Autodesk Inventor part; units mm, degrees
ref_plane "Work Plane1" through (29, 0, 0) normal (0, -1, 0) x (1, 0, 0)
ref_plane "YZ Plane" through (0, 0, 0) normal (1, 0, 0) x (0, 1, 0)
ref_plane "XZ Plane" through (0, 0, 0) normal (0, 1, 0) x (-1, 0, 0)
sketch "Skizze1" plane through (0, 0, 0) normal (0, 0, 1) x (1, 0, 0)
  line L0 (-2.3333, 0) -> (20, 0)
  line L1 (20, 0) -> (20, 5)
  line L2 (20, 5) -> (3.75, 5)
  line L3 (3.75, 5) -> (2.8297, 5)
  line L4 (2.8297, 5) -> (0, 5)
  line L5 (0, 5) -> (0, 8)
  line L6 (0, 8) -> (-10, 8)
  line L7 (-10, 8) -> (-10, 4.6188)
  line L8 (-10, 4.6188) -> (-5, 4.6188)
  line L9 (-5, 4.6188) -> (-2.3333, 0)
  line L10 (-16, 0) -> (26, 0)
  line L11 (0, -1.6) -> (0, 9.6)
  line L12 (3.75, 5) -> (0, 5) construction
  dimension "d1" = 16.25
  dimension "d2" = 0.9203
  dimension "d3" = 10
  dimension "d4" = 5
  dimension "d5" = 60
  dimension "d6" = 10
  dimension "d7" = 10
  dimension "d8" = 9.2376
  dimension "d9" = 16
  dimension "d26" = 20
revolve "Körper" add sketch "Skizze1" angle 360 about axis through (-2.3333, 0, 0) along (1, 0, 0)
sketch "Skizze2" plane through (-10, 0, 0) normal (-1, 0, 0) x (0, 0, 1)
  circle A0 centre (0, 0) radius 4.6188
  line L0 (0, -11.2) -> (0, 11.2)
  line L1 (-11.2, 0) -> (11.2, 0)
  line L2 (4.6188, 0) -> (2.3094, -4)
  line L3 (2.3094, -4) -> (-2.3094, -4)
  line L4 (-2.3094, -4) -> (-4.6188, 0)
  line L5 (-4.6188, 0) -> (-2.3094, 4)
  line L6 (-2.3094, 4) -> (2.3094, 4)
  line L7 (2.3094, 4) -> (4.6188, 0)
  point P0 (0, 0)
extrude "Loch" add sketch "Skizze2" against normal up to next contours L7 A0 | A0 L2 | L6 L0 A0 | A0 L0 L3 | L0 L6 A0 | A0 L3 L0 | L4 A0 | A0 L5
fillet "Rundung1" radius 1 1 edges at (-10, -8, 0)
thread "Gewinde"
chamfer "Fase1" distance 0.9202 distance2 0.9202 1 edges at (20, -5, 0) measured on face at (20, -0.8193, -0.3214)
ref_plane "Work Plane1" through (29, 0, 0) normal (0, -1, 0) x (1, 0, 0)
fillet "Fillet2" radius 0.1 1 edges at (0, -5, 0)
equation "\"d30\" = R"
equation "\"d17\" = RR"
equation "\"d13\" = GEL"
equation "\"d15\" = -0.5 * SPD + 0.5 * GD"
equation "\"d16\" = GUL"
equation "\"d1\" = GEL"
equation "\"d3\" = KOH"
equation "\"d4\" = INTI"
equation "\"d6\" = GD"
equation "\"d7\" = BDM"
equation "\"d8\" = 1.1547 * SW"
equation "\"d9\" = KOD"
equation "\"d26\" = NLG"
equation "\"GD\" = 10"
equation "\"NLG\" = 20"
equation "\"GEL\" = 16.25"
equation "\"KOD\" = 16"
equation "\"KOH\" = 10"
equation "\"INTI\" = 5"
equation "\"GAL\" = 0.61345 * PTC"
equation "\"GUL\" = 0.61345 * PTC"
equation "\"BDM\" = NND"
equation "\"SW\" = 8"
equation "\"RR\" = 1"
equation "\"SPD\" = NND - 1.2269 * PTC"
equation "\"R\" = 0.1"
equation "\"TOA\" = 30deg"
equation "\"GD1\" = THREADDIA - 1.2269 * PTC"
equation "\"FAWI\" = 45deg"
equation "\"PTC\" = 1.5"
equation "\"E0\" = 1.155 * SW"
properties part number "ISO 4762 - M10 x 20" material "Edelstahl, 440C"
Verification items for the finished model (mm, model axes). A direction names the side the tool comes from. Give positions to 0.01 mm unless a question says otherwise; leave off trailing zeros. Order: outer loops, then holes, each group sorted by start corner. A loop starts at its lowest first (then second) coordinate and runs counter-clockwise, first axis right, second up. Notation, with made-up numbers: M 42.25,64 L 61.25,64 A25 cw 61.25,78 Z; hole C -33,68 d4. An arc over 180 degrees is marked long. Answer as a JSON object with one key per item and string values. Group by question number.
1) Depth check by flat-ended pin: pin 1 Ø1.5 at (x, y) = (0, -4) entering from -Z; pin 2 Ø1.5 at (y, z) = (-6.5, -3.5) entering from +X; pin 3 Ø6 at (x, z) = (15.5, 4.5) entering from +Y. Enter the tip coordinate at first touch or a pass-through.
2) Mould release check, pull along Z, two halves, no side actions. Record for faces 1 (the face through (-7.359, -2.028, -3.448)), 2 (the face through (-7.36, -1.97, 3.48)), 3 (the face through (9.46, -1.08, 4.88)), 4 (the face through (20, 0, 0)): released by +Z, released by -Z, zero draft, split by the parting line, or undercut.
3) Access from +Z, -Z, +X, -X, +Y, -Y to the whole of each face (thin tool, end or side, straight path). Record for faces 5 (the face through (0, 5, -2)), 6 (the face through (-7.359, 2.028, 3.448)), 7 (the face through (-4.56, -1.73, 7.81)).
4) Cross-section at B-B (x = 12.75). Enter the section's corners in (y, z), then the cut area to 3 significant figures.
5) Cross-section at A-A (x = -7.25). Enter the section's corners in (y, z), then the cut area to 3 significant figures.
6) Scan lines: line 1 along X through (y, z) = (0.5, 6.25); line 2 along Y through (x, z) = (-5.25, -3.5); line 3 along Z through (x, y) = (-6.5, 6.25). Record each from-to range of solid material in increasing order. Write a range as [from, to].
Result sheet:
{
 "1": {"pin 1": "stops at z = -7.31", "pin 2": "stops at x = 0", "pin 3": "stops at y = 4.77"},
 "2": {"face 1": "undercut", "face 2": "undercut", "face 3": "split by the parting line", "face 4": "zero draft"},
 "3": {"face 5": "+X", "face 6": "-X", "face 7": "+X, -X"},
 "4": {"outline": "C 0,0 d10", "area": "78.5 mm2"},
 "5": {"outline": "C 0,0 d16; hole M -4,-2.31 L 0,-4.62 L 4,-2.31 L 4,2.31 L 0,4.62 L -4,2.31 Z", "area": "146 mm2"},
 "6": {"line 1": "x = [-10, 0]", "line 2": "y = [-7.19, -1.94], [1.94, 7.19]", "line 3": "z = [-4.99, 4.99]"}
}
